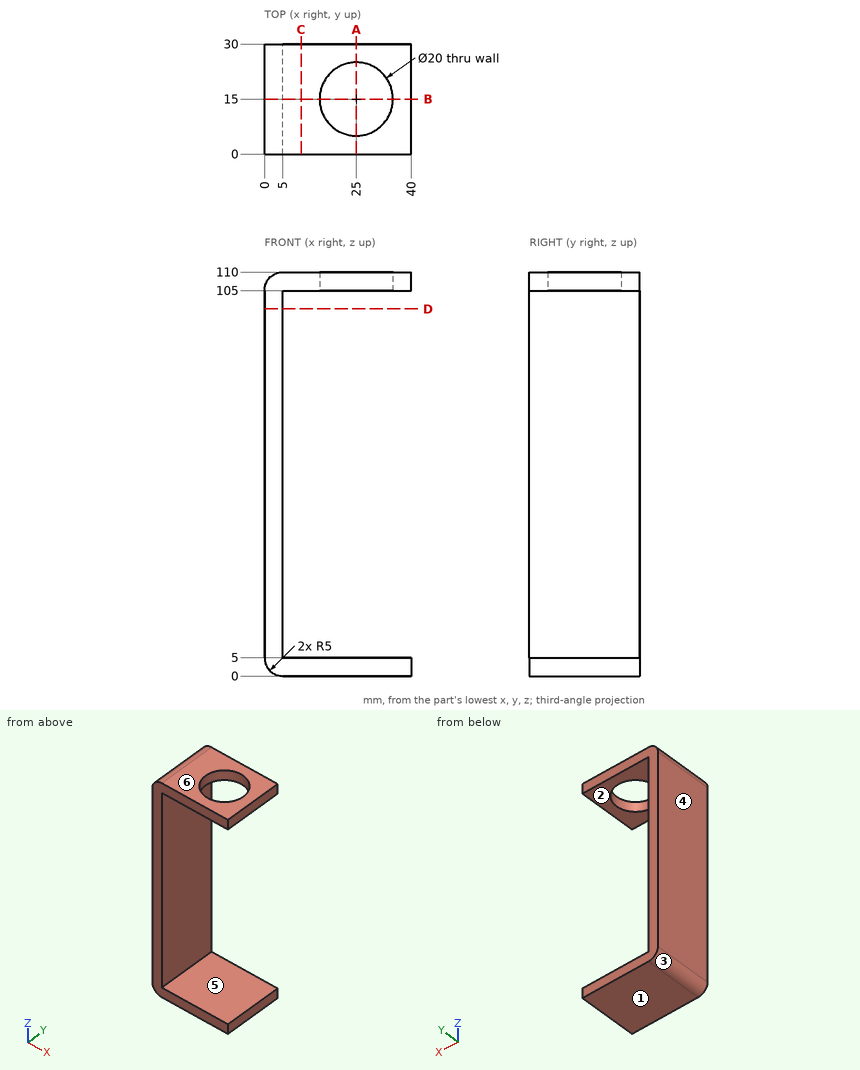
For this review, use the dimensioned drawing (mm, ordinates from the lowest corner) and the shaded views. A direction names the side the tool comes from. Coordinates: 2 decimals unless noted, no trailing zeros. Loops run counter-clockwise (first coordinate to the right, second up) from the corner with the lowest first, then second, coordinate; pieces in that order, holes last. Notation, with made-up numbers: (4, -30) -> (31, -30) arc R22 cw to (31, 1) -> close; hole circle Ø9 at (-28.5, 49). An arc over 180 degrees is marked (long way). Use a Markdown table: item, result. Add a question column.
Item 1: Clearance check with flat-ended pins moving along their axes: P1, Ø9, axis at x = 25.5, y = 15.5, coming from the +Z side; P2, Ø1, axis at y = 6, z = 58, coming from the +X side. State where each tip first meets the part, or that it passes through.
Item 2: Machinability: for the marked faces 1 and 2, which of the approach directions +Z, -Z, +X, -X, +Y, -Y give a long, thin tool a straight path to every point of the face, cutting with its end or side? Answer none if there is none.
Item 3: We need section B-B, the plane y = 15. Write out the cut boundary in (x, z), and give its area (3 significant figures).
Item 4: We need section C-C, the plane x = 10. Write out the cut boundary in (y, z), and give its area (3 significant figures).
Item 5: The part is to be moulded in two halves that separate along Z. For the marked faces 3, 4, 5 and 6, say which applies: +Z half, -Z half, draft (parallel to the pull), parting line (faces both ways), or undercut.
Item 6: We need section A-A, the plane x = 25. Write out the cut boundary in (y, z).
Item 7: Wall thickness on L1, parallel to Y at x = 25, z = 107; L2, parallel to Z at x = 31, y = 6.75; L3, parallel to X at y = 27, z = 34: over which ranges is each line inside the solid? List them lowest first. Write a range as from..to.
Item 8: We need section D-D, the plane z = 100. Write out the cut boundary in (x, y).
Numbers:
| question | item | result |
|---|---|---|
| 1 | P1 | stops at z = 5 |
| 1 | P2 | stops at x = 5 |
| 2 | face 1 | -Z, +X, -X, +Y, -Y |
| 2 | face 2 | +X, +Y, -Y |
| 3 | outline | (0, 5) arc R5 ccw to (5, 0) -> (40, 0) -> (40, 5) -> (5, 5) -> (5, 105) -> (15, 105) -> (15, 110) -> (5, 110) arc R5 ccw to (0, 105) -> close; (35, 105) -> (40, 105) -> (40, 110) -> (35, 110) -> close |
| 3 | area | 789 mm^2 |
| 4 | outline | (0, 0) -> (30, 0) -> (30, 5) -> (0, 5) -> close; (0, 105) -> (30, 105) -> (30, 110) -> (0, 110) -> close |
| 4 | area | 300 mm^2 |
| 5 | face 3 | -Z half |
| 5 | face 4 | draft |
| 5 | face 5 | undercut |
| 5 | face 6 | +Z half |
| 6 | outline | (0, 0) -> (30, 0) -> (30, 5) -> (0, 5) -> close; (0, 105) -> (5, 105) -> (5, 110) -> (0, 110) -> close; (25, 105) -> (30, 105) -> (30, 110) -> (25, 110) -> close |
| 7 | L1 | y = 0..5, 25..30 |
| 7 | L2 | z = 0..5, 105..110 |
| 7 | L3 | x = 0..5 |
| 8 | outline | (0, 0) -> (5, 0) -> (5, 30) -> (0, 30) -> close |
